CAD build for the part. Positions are in the model's coordinates, mm. Face numbers are marked on the shaded views. A direction names the side the tool comes from. Coordinates: 2 decimals unless noted, no trailing zeros. Order: outer loops, then holes, each group sorted by start corner. A loop starts at its lowest first (then second) coordinate and runs counter-clockwise, first axis right, second up. Notation, with made-up numbers: M 46.5,83 L 85.5,83 A26 ccw 85.5,100 Z; hole C -22.5,13 d8. An arc over 180 degrees is marked long. Write item = value, one per line. Start each with the question number.
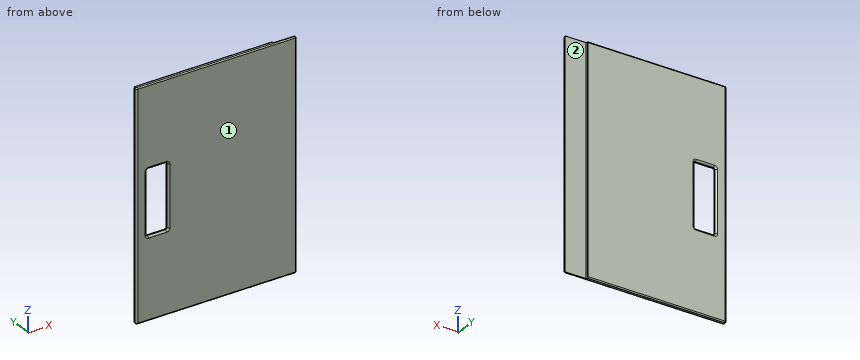
Autodesk Inventor part; units mm, degrees
ref_plane "YZ Plane" through (0, 0, 0) normal (1, 0, 0) x (0, 1, 0)
ref_plane "XZ Plane" through (0, 0, 0) normal (0, 1, 0) x (-1, 0, 0)
ref_plane "XY Plane" through (0, 0, 0) normal (0, 0, 1) x (1, 0, 0)
sketch "Sketch1" plane through (0, 0, 0) normal (0, 1, 0) x (-1, 0, 0)
  line L0 (0, 0) -> (300, 0)
  line L1 (300, 0) -> (300, -420)
  line L2 (300, -420) -> (0, -420)
  line L3 (0, -420) -> (0, 0)
  line L4 (240, -150) -> (280, -150)
  line L5 (280, -150) -> (280, -270)
  line L6 (280, -270) -> (240, -270)
  line L7 (240, -270) -> (240, -150)
  line L8 (240, -150) -> (280, -270) construction
  line L9 (280, -150) -> (240, -270) construction
  dimension "d0" = 300
  dimension "d1" = 420
  dimension "d5" = 40
  dimension "d6" = 120
extrude "Extrusion1" add sketch "Sketch1" along normal blind 8
sketch "Sketch2" plane through (0, 0, 0) normal (1, 0, 0) x (0, 0, -1)
  line L0 (150, 0) -> (270, 0)
  line L1 (210, 0) -> (210, 4)
  line L2 (420, 0) -> (420, 8)
  line L3 (0, 4.5) -> (420, 4.5)
  line L4 (420, 4.5) -> (420, 3.5)
  line L5 (420, 3.5) -> (0, 3.5)
  line L6 (0, 3.5) -> (0, 4.5)
  line L7 (0, 4.5) -> (420, 3.5) construction
  line L8 (420, 4.5) -> (0, 3.5) construction
  line L9 (0, 0) -> (0, 8)
  line L10 (420, 3.5) -> (0, 3.5)
  line L11 (0, 3.5) -> (0, 8)
  line L12 (0, 8) -> (420, 8)
  line L13 (420, 8) -> (420, 3.5)
  dimension "d7" = 4
  dimension "d8" = 1
extrude "Extrusion2" cut sketch "Sketch2" against normal blind 40
fillet "Fillet1" radius 3.1 14 edges at (-300, 8, -210) (-300, 0, -210) (-280, 8, -210) (-260, 8, -270) (-240, 8, -210) (-280, 0, -210) (-260, 0, -270) (-280, 4, -270) (-240, 4, -270) (-240, 4, -150) (-260, 0, -150) (-260, 8, -150) (-280, 4, -150) (-240, 0, -210)
fillet "Fillet2" radius 2 11 edges at (-299.092, 7.092, 0) (-300, 4, 0) (-299.092, 0.908, 0) (-148.45, 0, 0) (-168.45, 8, 0) (-299.092, 7.092, -420) (-300, 4, -420) (-299.092, 0.908, -420) (-148.45, 0, -420) (-168.45, 8, -420) (0, 0, -210)
fillet "Fillet3" radius 0.3 8 edges at (-40, 7.4142, -419.4142) (-40, 4.75, -420) (-40, 7.4142, -0.5858) (-40, 4.75, 0) (-40, 8, -210) (-20, 3.5, -420) (0, 3.5, -210) (-20, 3.5, 0)
fillet "Fillet4" radius 2 6 edges at (-0.0879, 3.4121, -0.0879) (-0.5858, 0.5858, -0.5858) (0, 2.6, 0) (-0.0879, 3.4121, -419.9121) (-0.5858, 0.5858, -419.4142) (0, 2.6, -420)
properties part number "RightFlap"
1. Flat gauge pin, fed straight in: pin 1 (2 mm diameter, centred on y = 5.5, z = -139, fed in from +X). Where does the tip first touch, or does it go through?
2. 3-axis set-ups, long thin cutter, end or side, ignore diameter. For the marked faces 1 and 2: which of +Z, -Z, +X, -X, +Y, -Y reach the whole face in a straight line?
3. Probe L1, parallel to X at y = 4.5, z = -206; L2, parallel to Y at x = -16, z = -284.5; L3, parallel to Z at x = -239, y = 7. List the from-to ranges inside material, lowest first.
4. Slice it at A-A (z = -172). Write the cut outline in (x, y).
Calculated:
q1.pin_1 = -40
q2.face_1 = +Z, -Z, +X, -X, -Y
q2.face_2 = +Z, -Z, +X, +Y
q3.L1 = -300 to -280, -240 to -40
q3.L2 = 0 to 3.5
q3.L3 = -419.73 to -0.27
q4.outline = M -300,3.1 A3.1 ccw -296.9,0 L -283.1,0 A3.1 ccw -280,3.1 L -280,4.9 A3.1 ccw -283.1,8 L -296.9,8 A3.1 ccw -300,4.9 Z; M -240,3.1 A3.1 ccw -236.9,0 L -2,0 A2 ccw 0,2 L 0,3.2 A0.3 ccw -0.3,3.5 L -40,3.5 L -40,7.7 A0.3 ccw -40.3,8 L -236.9,8 A3.1 ccw -240,4.9 Z
